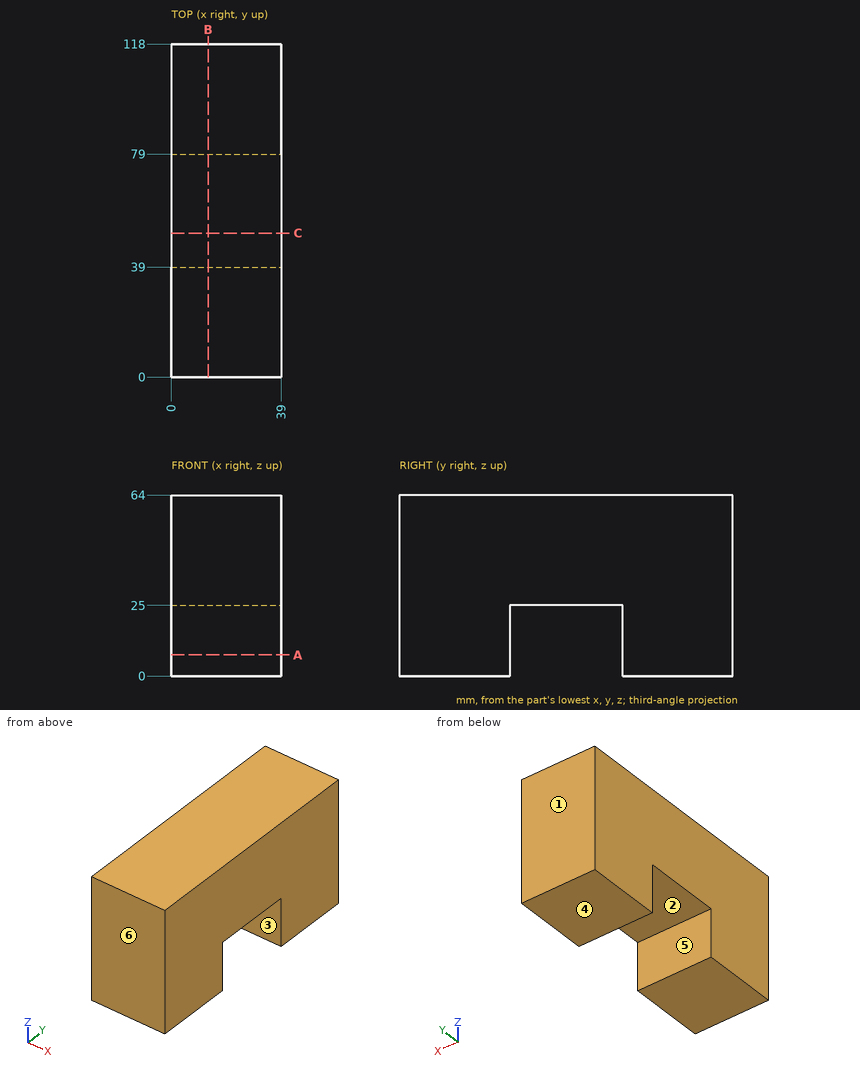
Geometry: see drawing. Coordinates: mm, zero at the bounding-box minimum. A direction names the side the tool comes from. Give positions to 0.01 mm unless a question says otherwise; leave off trailing zeros. Order: outer loops, then holes, each group sorted by start corner. A loop starts at its lowest first (then second) coordinate and runs counter-clockwise, first axis right, second up. Notation, with made-up numbers: (71.25, -21.5) -> (80.25, -21.5) arc R21 cw to (80.25, -13.5) -> close; hole circle Ø5 at (75, -21.75). An arc over 180 degrees is marked (long way). Write item = value, one per line.
Q1. Pull-direction query (Y, two-part tool) for the marked faces 1, 2, 3 and 4; classes: released by +Y, released by -Y, zero draft, split by the parting line, or undercut.
Data:
face_1 = released by +Y
face_2 = undercut
face_3 = undercut
face_4 = zero draft
Q2. Material intervals for line 1 (Y direction, x = 24.5, z = 13); line 2 (Z direction, x = 34.5, y = 71), sorted ascending. Write a range as from..to.
Data:
line_1 = 0..39, 79..118
line_2 = 25..64
Q3. Cut plane C-C, the plane y = 51. Output: boundary loops of the cut face in (x, z).
Data:
outline = (0, 25) -> (39, 25) -> (39, 64) -> (0, 64) -> close
Q4. Set-up query: the marked faces 5 and 6. Return all of +Z, -Z, +X, -X, +Y, -Y with unobstructed straight access to the full face (end or side cutting, diameter ignored); none if empty.
Data:
face_5 = -Z, +X, -X
face_6 = +Z, -Z, +X, -X, -Y
Q5. Cut plane A-A, the plane z = 7.5. Output: boundary loops of the cut face in (x, y).
Data:
outline = (0, 0) -> (39, 0) -> (39, 39) -> (0, 39) -> close; (0, 79) -> (39, 79) -> (39, 118) -> (0, 118) -> close
Q6. Pin query (flat end, axial travel): pin 1 (19.5 mm diameter, centred on x = 11, y = 59, fed in from -Z). Return the tip coordinate at first contact, or that it passes through.
Data:
pin_1 = 25
Q7. Cut plane B-B, the plane x = 13. Output: boundary loops of the cut face in (y, z), and give its area (3 significant figures).
Data:
outline = (0, 0) -> (39, 0) -> (39, 25) -> (79, 25) -> (79, 0) -> (118, 0) -> (118, 64) -> (0, 64) -> close
area = 6,550 mm^2
